Geometry check sheet. Reference: the model listing, model coordinates, mm. Give positions to 0.01 mm unless a question says otherwise; leave off trailing zeros. Write each loop counter-clockwise with the first axis right and the second up, starting at its lowest first coordinate (ties: lowest second). Pieces come first, ordered by that corner, then holes.
(1) Depth check by flat-ended pin: P1, Ø1.5, axis at y = 1.5, z = -107, coming from the +X side; P2, Ø0.9, axis at x = 9, y = 1, coming from the +Z side; P3, Ø1.5, axis at y = 2, z = -157.5, coming from the -X side. Enter the tip coordinate at first touch or a pass-through.
(2) Cross-section at B-B (z = -155). Record the boundary of the cut face in (x, y).
(3) Cross-section at D-D (y = 1.35). Count the separate pieces of the cut face and the enclosed holes in it, and give its area (3 significant figures).
(4) Cross-section at A-A (x = 11.5). Record the boundary of the cut face in (y, z).
(5) Cross-section at C-C (z = 47). Record the boundary of the cut face in (x, y), and give its area (3 significant figures).
(6) Thickness scan on line 1 along Z through (x, y) = (35, 1.85); line 2 along Z through (x, y) = (-4, 1.1); line 3 along Z through (x, y) = (-28, 1.65). Record the ranges inside material, lowest first.
```python
from build123d import *

# Parameters (mm, degrees)
ESQUISSE1_W             = 60.5
ESQUISSE1_H             = 60
BOSS_EXTRU_1_DEPTH      = 3
ESQUISSE2_R             = 2.1
ENL_V_MAT_EXTRU_1_DEPTH = 275.531688146
ESQUISSE6_W             = 4
ESQUISSE6_H             = 8
ENL_V_MAT_EXTRU_2_DEPTH = 275.531688146


with BuildPart() as part:
    # Esquisse1 → Boss.-Extru.1 (new body)
    with BuildSketch(Plane(origin=(0, 0, 0), x_dir=(1, 0, 0), z_dir=(0, 1, 0))):
        Polygon((-147.224318643, -136.961524227), (-103.923048454, -111.961524227), (103.923048454, -111.961524227), (147.224318643, -136.961524227), (192.224318643, -59.019237886), (148.923048454, -34.019237886), (45, 145.980762114), (45, 195.980762114), (-45, 195.980762114), (-45, 145.980762114), (-148.923048454, -34.019237886), (-192.224318643, -59.019237886), align=None)
        Polygon((-137.278810568, -114.187649521), (-167.528810568, -61.793112592), (-115.567286341, -31.793112592), (-85.317286341, -84.187649521), align=None, mode=Mode.SUBTRACT)
        Polygon((167.528810568, -61.793112592), (137.278810568, -114.187649521), (85.317286341, -84.187649521), (115.567286341, -31.793112592), align=None, mode=Mode.SUBTRACT)
        with Locations((0, 145.980762114)):
            Rectangle(ESQUISSE1_W, ESQUISSE1_H, mode=Mode.SUBTRACT)
    extrude(amount=BOSS_EXTRU_1_DEPTH)

    # Esquisse2 → Enlèv. mat.-Extru.1 (cut, through all)
    with BuildSketch(Plane(origin=(0, 3, 0), x_dir=(1, 0, 0), z_dir=(0, 1, 0))):
        with Locations(Location((-35, 185.980762114, 0), (0, 0, 270))):
            Circle(ESQUISSE2_R)
        with Locations(Location((35, 185.980762114, 0), (0, 0, 90))):
            Circle(ESQUISSE2_R)
        with Locations(Location((-143.564064605, -123.301270189, 0), (0, 0, 270))):
            Circle(ESQUISSE2_R)
        with Locations(Location((-178.564064605, -62.679491924, 0), (0, 0, 90))):
            Circle(ESQUISSE2_R)
        with Locations(Location((178.564064606, -62.679491924, 0), (0, 0, 270))):
            Circle(ESQUISSE2_R)
        with Locations(Location((143.564064606, -123.301270189, 0), (0, 0, 90))):
            Circle(ESQUISSE2_R)
        with Locations(Location((88.301270189, 50.980762114, 0), (0, 0, 270))):
            Circle(ESQUISSE2_R)
        with Locations(Location((0, -101.961524227, 0), (0, 0, 270))):
            Circle(ESQUISSE2_R)
        with Locations(Location((-88.301270189, 50.980762114, 0), (0, 0, 270))):
            Circle(ESQUISSE2_R)
    extrude(amount=-ENL_V_MAT_EXTRU_1_DEPTH, mode=Mode.SUBTRACT)

    # Esquisse6 → Enlèv. mat.-Extru.2 (cut, through all)
    with BuildSketch(Plane(origin=(0, 3, 0), x_dir=(1, 0, 0), z_dir=(0, 1, 0))):
        with Locations((-35, 111.980762114)):
            Rectangle(ESQUISSE6_W, ESQUISSE6_H)
        Polygon((-37, 105.980762114), (-37, 103.980762114), (-33, 103.980762114), (-33, 105.980762114), (-33, 107.980762114), (-37, 107.980762114), align=None)
        Polygon((-45, 107.980762114), (-45, 103.980762114), (-37, 103.980762114), (-37, 105.980762114), (-37, 107.980762114), align=None)
        Polygon((-33, 105.980762114), (-33, 103.980762114), (-25, 103.980762114), (-25, 107.980762114), (-33, 107.980762114), align=None)
        with Locations((-35, 99.980762114)):
            Rectangle(ESQUISSE6_W, ESQUISSE6_H)
        Polygon((33, 105.980762114), (33, 107.980762114), (25, 107.980762114), (25, 103.980762114), (33, 103.980762114), align=None)
        with Locations((35, 111.980762114)):
            Rectangle(ESQUISSE6_W, ESQUISSE6_H)
        Polygon((37, 105.980762114), (37, 107.980762114), (33, 107.980762114), (33, 105.980762114), (33, 103.980762114), (37, 103.980762114), align=None)
        Polygon((45, 103.980762114), (45, 107.980762114), (37, 107.980762114), (37, 105.980762114), (37, 103.980762114), align=None)
        with Locations((35, 99.980762114)):
            Rectangle(ESQUISSE6_W, ESQUISSE6_H)
        Polygon((116.01408311, -15.019237886), (112.549981495, -13.019237886), (108.549981495, -19.947441117), (110.282032303, -20.947441117), (112.01408311, -21.947441117), align=None)
        Polygon((110.282032303, -20.947441117), (108.549981495, -19.947441117), (106.549981495, -23.411542732), (108.282032303, -24.411542732), (110.01408311, -25.411542732), (112.01408311, -21.947441117), align=None)
        Polygon((108.549981495, -19.947441117), (101.621778265, -15.947441117), (99.621778265, -19.411542732), (106.549981495, -23.411542732), align=None)
        Polygon((108.282032303, -24.411542732), (106.549981495, -23.411542732), (102.549981495, -30.339745962), (106.01408311, -32.339745962), (110.01408311, -25.411542732), align=None)
        Polygon((118.942286341, -25.947441117), (112.01408311, -21.947441117), (110.01408311, -25.411542732), (116.942286341, -29.411542732), align=None)
        Polygon((64.621778265, -80.033320997), (71.549981495, -84.033320997), (73.549981495, -80.569219382), (66.621778265, -76.569219382), align=None)
        Polygon((75.282032303, -81.569219382), (77.01408311, -82.569219382), (81.01408311, -75.641016151), (77.549981495, -73.641016151), (73.549981495, -80.569219382), align=None)
        Polygon((73.282032303, -85.033320997), (75.01408311, -86.033320997), (77.01408311, -82.569219382), (75.282032303, -81.569219382), (73.549981495, -80.569219382), (71.549981495, -84.033320997), align=None)
        Polygon((77.01408311, -82.569219382), (75.01408311, -86.033320997), (81.942286341, -90.033320997), (83.942286341, -86.569219382), align=None)
        Polygon((67.549981495, -90.961524227), (71.01408311, -92.961524227), (75.01408311, -86.033320997), (73.282032303, -85.033320997), (71.549981495, -84.033320997), align=None)
        Polygon((-75.282032303, -81.569219382), (-73.549981495, -80.569219382), (-77.549981495, -73.641016151), (-81.01408311, -75.641016151), (-77.01408311, -82.569219382), align=None)
        Polygon((-81.942286341, -90.033320997), (-75.01408311, -86.033320997), (-77.01408311, -82.569219382), (-83.942286341, -86.569219382), align=None)
        Polygon((-71.01408311, -92.961524227), (-67.549981495, -90.961524227), (-71.549981495, -84.033320997), (-73.282032303, -85.033320997), (-75.01408311, -86.033320997), align=None)
        Polygon((-71.549981495, -84.033320997), (-64.621778265, -80.033320997), (-66.621778265, -76.569219382), (-73.549981495, -80.569219382), align=None)
        Polygon((-110.01408311, -25.411542732), (-112.01408311, -21.947441117), (-118.942286341, -25.947441117), (-116.942286341, -29.411542732), align=None)
        Polygon((-112.549981495, -13.019237886), (-116.01408311, -15.019237886), (-112.01408311, -21.947441117), (-110.282032303, -20.947441117), (-108.549981495, -19.947441117), align=None)
        Polygon((-110.282032303, -20.947441117), (-112.01408311, -21.947441117), (-110.01408311, -25.411542732), (-108.282032303, -24.411542732), (-106.549981495, -23.411542732), (-108.549981495, -19.947441117), align=None)
        Polygon((-101.621778265, -15.947441117), (-108.549981495, -19.947441117), (-106.549981495, -23.411542732), (-99.621778265, -19.411542732), align=None)
        Polygon((-108.282032303, -24.411542732), (-110.01408311, -25.411542732), (-106.01408311, -32.339745962), (-102.549981495, -30.339745962), (-106.549981495, -23.411542732), align=None)
        Polygon((-73.282032303, -85.033320997), (-71.549981495, -84.033320997), (-73.549981495, -80.569219382), (-75.282032303, -81.569219382), (-77.01408311, -82.569219382), (-75.01408311, -86.033320997), align=None)
    extrude(amount=-ENL_V_MAT_EXTRU_2_DEPTH, mode=Mode.SUBTRACT)


solid = part.part
```
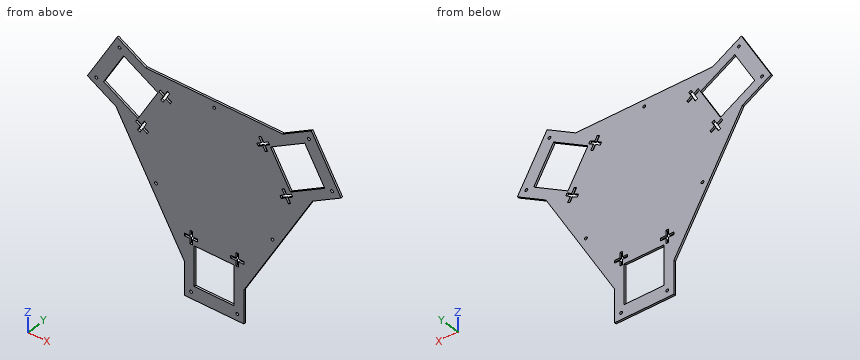
Reply:
1. P1: stops at x = 67.94
1. P2: stops at z = 111.96
1. P3: stops at x = -45
2. outline: (-45, 0) - (-30.25, 0) - (-30.25, 3) - (-45, 3) - close; (30.25, 0) - (45, 0) - (45, 3) - (30.25, 3) - close
3. separate pieces: 1
3. enclosed holes: 18
3. area: 56,200 mm2
4. outline: (0, -195.98) - (3, -195.98) - (3, -175.98) - (0, -175.98) - close; (0, -115.98) - (3, -115.98) - (3, 111.96) - (0, 111.96) - close
5. outline: (-171.41, 0) - (-141.91, 0) - (-141.91, 3) - (-171.41, 3) - close; (-106.79, 0) - (106.79, 0) - (106.79, 3) - (-106.79, 3) - close; (141.91, 0) - (171.41, 0) - (171.41, 3) - (141.91, 3) - close
5. area: 818 mm2
6. line 1: z = -195.98 to -188.08, -183.88 to -115.98, -95.98 to 111.96
6. line 2: z = -195.98 to -175.98, -115.98 to 111.96
6. line 3: z = -195.98 to -175.98, -115.98 to -107.98, -103.98 to 111.96
